Geometry check sheet. Reference: the model listing, model coordinates, mm. Round coordinates to 2 decimals unless told otherwise and drop trailing zeros. Order: outer loops, then holes, each group sorted by start corner. A loop starts at its lowest first (then second) coordinate and runs counter-clockwise, first axis right, second up. Notation, with made-up numbers: (43, 2.5) - (73, 2.5) arc R20 ccw to (73, 10.5) - close; hole circle Ø2 at (-30, -34). An arc over 180 degrees is marked (long way). Return JSON: item names as keys, results as strings. Group by question number.
Q1. Gauge pin test, flat ends, axial feed: pin 1 Ø1 at (x, z) = (15, -5) entering from +Y; pin 2 Ø6 at (x, y) = (-35, 17) entering from -Z; pin 3 Ø1.5 at (y, z) = (47.5, 2) entering from +X. Record the tip position at first contact, or that the pin passes through.
Q2. Sectioned sample at A-A, the plane y = 43. Record the cut outline in (x, z), then the cut area to 3 significant figures.
Q3. Sectioned sample at C-C, the plane y = 58.5. Record the cut outline in (x, z), then the cut area to 3 significant figures.
Q4. Sectioned sample at B-B, the plane x = 28. Record the cut outline in (y, z), then the cut area to 3 significant figures.
Q5. Material ranges on line 1 along Z through (x, y) = (14.5, 60); line 2 along Z through (x, y) = (18, 26); line 3 along Y through (x, z) = (29, -4), recorded low to high.
```python
from build123d import *

# Parameters (mm, degrees)
F1_DEPTH = 6.35
F3_DEPTH = 25.4
F4_R     = 3.81
F7_R     = 5.08


with BuildPart() as f1:
    # F0 (on Top) → F1 (new body, symmetric)
    with BuildSketch(Plane.XY):
        with BuildLine():
            Line((-63.5, 0), (63.5, 0))
            ThreePointArc((63.5, 0), (0, 63.5), (-63.5, 0))
        make_face()
    extrude(amount=F1_DEPTH, both=True)

    # F2 (on Top) → F3 (cut)
    with BuildSketch(Plane.XY):
        with BuildLine():
            Line((-50.2836502119, 7.2245775906), (50.2836502119, 7.2245775906))
            ThreePointArc((50.2836502119, 7.2245775906), (0, 50.8), (-50.2836502119, 7.2245775906))
        make_face()
    extrude(amount=-F3_DEPTH, mode=Mode.SUBTRACT)

    # F6: sweep along a path in F5
    with BuildLine(Plane.YZ) as f6_path:
        Line((25.5370624363, 0), (6.1716223136, -26.4036767185))
    # F4 (on Top) → F6 (sweep, cut)
    with BuildSketch(Plane.XY):
        with Locations((0, 25.4)):
            Circle(F4_R)
    sweep(path=f6_path.line, mode=Mode.SUBTRACT)

    # F8: sweep along a path in F5
    with BuildLine(Plane.YZ) as f8_path:
        Line((25.5370624363, 0), (6.1716223136, -26.4036767185))
    # F7 (on Top) → F8 (sweep)
    with BuildSketch(Plane.XY):
        with Locations((0, 25.4)):
            Circle(F7_R)
    sweep(path=f8_path.line)


solid = f1.part
```
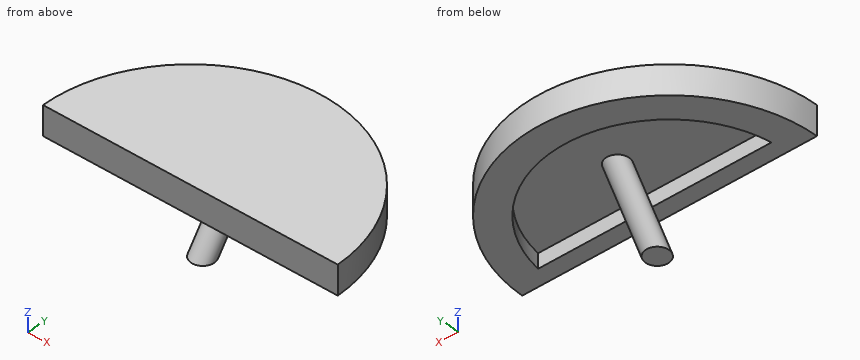
Reply:
{
 "1": {"pin 1": "y = 61.82", "pin 2": "z = 0", "pin 3": "x = 42.97"},
 "2": {"outline": "(-46.73, -6.35) - (-27.05, -6.35) - (-27.05, 0) - (27.05, 0) - (27.05, -6.35) - (46.73, -6.35) - (46.73, 6.35) - (-46.73, 6.35) - close", "area": "843 mm^2"},
 "3": {"outline": "(-24.7, -6.35) - (24.7, -6.35) - (24.7, 6.35) - (-24.7, 6.35) - close", "area": "627 mm^2"},
 "4": {"outline": "(0, -6.35) - (7.22, -6.35) - (7.22, 0) - (42.39, 0) - (42.39, -6.35) - (56.99, -6.35) - (56.99, 6.35) - (0, 6.35) - close", "area": "501 mm^2"},
 "5": {"line 1": "-6.35 to 6.35", "line 2": "0 to 6.35", "line 3": "0 to 7.22, 41.71 to 56.49"}
}
